Source: CAD feature listing. Evaluate the final solid. Frame: model axes, mm. A direction names the side the tool comes from. Round coordinates to 2 decimals unless told otherwise and drop trailing zeros. Order: outer loops, then holes, each group sorted by start corner. A loop starts at its lowest first (then second) coordinate and runs counter-clockwise, first axis right, second up. Notation, with made-up numbers: (14.25, 58.25) -> (41.25, 58.25) arc R17 ccw to (41.25, 64.25) -> close; hole circle Ø9 at (28.25, 46.5). An arc over 180 degrees is marked (long way). Answer as CSV lines item,"result".
from build123d import *

# Parameters (mm, degrees)
IZIM1_R                                 = 2.5
IZIM1_R_2                               = 2
Y_KSEKLIK_EKSTR_ZYON1_DEPTH             = 5
IZIM2_R                                 = 2
IZIM2_R_2                               = 1.5
Y_KSEKLIK_EKSTR_ZYON2_DEPTH             = 35
Y_KSEKLIK_EKSTR_ZYON2_DIRECTION_2_REACH = 7
IZIM3_R                                 = 2.5
IZIM3_R_2                               = 2
Y_KSEKLIK_EKSTR_ZYON3_DEPTH             = 10


with BuildPart() as part:
    # Çizim1 → Yükseklik-Ekstrüzyon1 (new body, symmetric)
    with BuildSketch(Plane.XY):
        Circle(IZIM1_R)
        Circle(IZIM1_R_2, mode=Mode.SUBTRACT)
    extrude(amount=Y_KSEKLIK_EKSTR_ZYON1_DEPTH, both=True)

    # Çizim2 → Yükseklik-Ekstrüzyon2 (add)
    with BuildSketch(Plane(origin=(2.5, 0, 0), x_dir=(0, 0, -1), z_dir=(1, 0, 0))):
        Circle(IZIM2_R)
        Circle(IZIM2_R_2, mode=Mode.SUBTRACT)
    extrude(amount=Y_KSEKLIK_EKSTR_ZYON2_DEPTH)

    # Çizim2 → Yükseklik-Ekstrüzyon2 direction 2 (add, up to next)
    with BuildSketch(Plane(origin=(2.5, 0, 0), x_dir=(0, 0, -1), z_dir=(1, 0, 0)), mode=Mode.PRIVATE) as y_kseklik_ekstr_zyon2_direction_2_sk1:
        Circle(IZIM2_R)
        Circle(IZIM2_R_2, mode=Mode.SUBTRACT)
    y_kseklik_ekstr_zyon2_direction_2_tool1 = extrude(y_kseklik_ekstr_zyon2_direction_2_sk1.sketch, amount=-Y_KSEKLIK_EKSTR_ZYON2_DIRECTION_2_REACH, mode=Mode.PRIVATE) - part.part
    add(y_kseklik_ekstr_zyon2_direction_2_tool1.solids().sort_by_distance((2.5, 0, 1.943431))[0])
    add(y_kseklik_ekstr_zyon2_direction_2_tool1.solids().sort_by_distance((2.5, 0, 1.943431))[1])

    # Çizim3 → Yükseklik-Ekstrüzyon3 (add)
    with BuildSketch(Plane(origin=(32.997737042, 0, 0), x_dir=(0, 0, -1), z_dir=(1, 0, 0))):
        Circle(IZIM3_R)
        Circle(IZIM3_R_2, mode=Mode.SUBTRACT)
    extrude(amount=-Y_KSEKLIK_EKSTR_ZYON3_DEPTH)


solid = part.part
1. Section query D-D on z = 3.75. Return loops of the section in (x, y).
Results below:
outline,"circle Ø5 at (0, 0); hole circle Ø4 at (0, 0)"
2. Pin query (flat end, axial travel): pin 1 (1 mm diameter, centred on x = 10, y = 0, fed in from +Z); pin 2 (3 mm diameter, centred on y = 1.5, z = -0.5, fed in from -X); pin 3 (4 mm diameter, centred on x = 3, z = -0.5, fed in from +Y); pin 4 (2.5 mm diameter, centred on x = 0, y = 0, fed in from -Z). Return the tip coordinate at first contact, or that it passes through.
Results below:
pin 1,"z = 2"
pin 2,"x = -2.5"
pin 3,"y = 2.29"
pin 4,"through"
3. Reachability of faces 4 (the flat face through (-1, 2, 5)), 5 (the cylindrical face through (28.07, -2.44, 0.54)), 6 (the flat face through (22.998, 2, 1)) from +Z, -Z, +X, -X, +Y, -Y: full face, straight path, thin tool, end or side. Return the list, or none.
Results below:
face 4,"+Z, +X, -X, +Y, -Y"
face 5,"+X"
face 6,"none"
4. Line query: L1, parallel to Z at x = 18, y = -0.1; L2, parallel to Y at x = 0, z = 2. Output: solid intervals per line, ascending. Write a range as [from, to].
Results below:
L1,"[-2, -1.5], [1.5, 2]"
L2,"[-2.5, -2], [2, 2.5]"
5. Section query C-C on x = 23.5. Return loops of the section in (y, z), and give its area (3 significant figures).
Results below:
outline,"circle Ø5 at (0, 0); hole circle Ø3 at (0, 0)"
area,"12.6 mm2"
6. Mould query, pull axis X, two halves, no side actions, for faces 1 (the flat face through (32.998, 2, 1)), 2 (the cylindrical face through (0, -2, 0)), 3 (the flat face through (-1, 2, -5)). Classes: released by +X, released by -X, zero draft, split by the parting line, or undercut.
Results below:
face 1,"released by +X"
face 2,"undercut"
face 3,"zero draft"
7. Section query A-A on z = 0. Return loops of the section in (x, y).
Results below:
outline,"(1.5, -2) -> (23, -2) -> (23, -2.5) -> (33, -2.5) -> (33, -2) -> (37.5, -2) -> (37.5, -1.5) -> (2, -1.5) arc R2.5 ccw to (2, 1.5) -> (37.5, 1.5) -> (37.5, 2) -> (33, 2) -> (33, 2.5) -> (23, 2.5) -> (23, 2) -> (1.5, 2) arc R2.5 ccw (long way) to start; hole circle Ø4 at (0, 0)"
8. Section query B-B on x = 0. Return loops of the section in (y, z).
Results below:
outline,"(-2.5, -5) -> (-2, -5) -> (-2, 5) -> (-2.5, 5) -> close; (2, -5) -> (2.5, -5) -> (2.5, 5) -> (2, 5) -> close"
